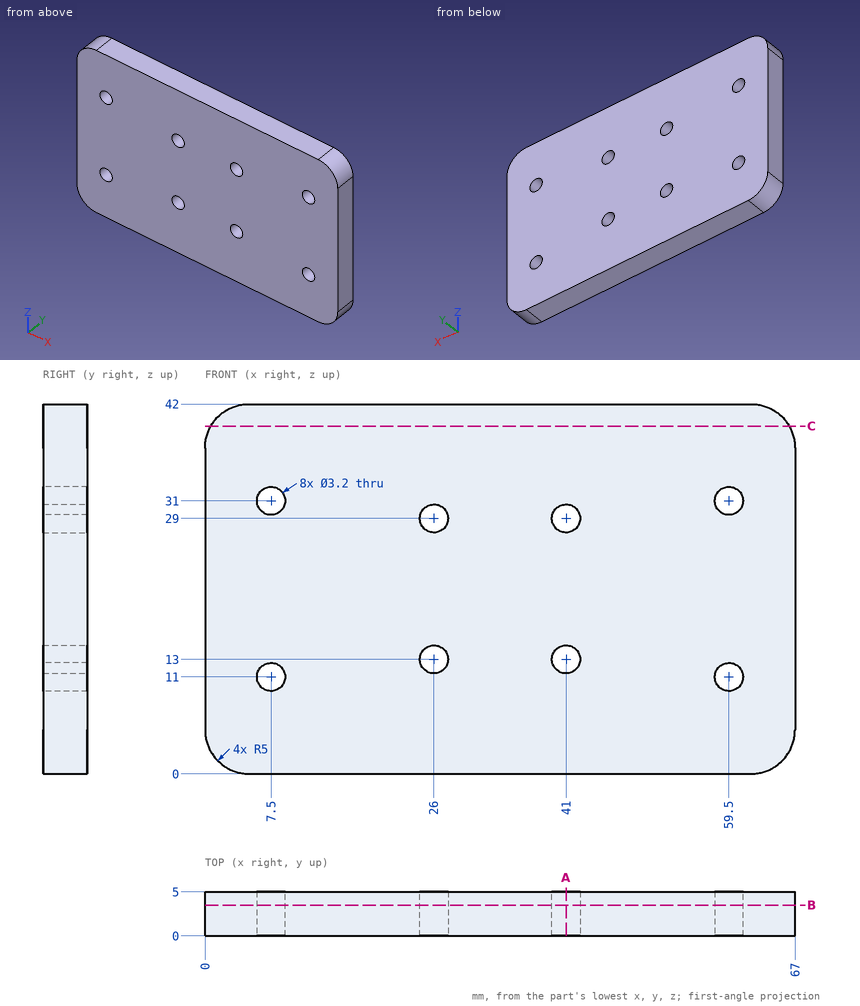
Study the drawing (mm; zero at the part's minimum x, y, z) and answer. Give positions to 0.01 mm unless a question says otherwise; leave off trailing zeros. Order: outer loops, then holes, each group sorted by start corner. A loop starts at its lowest first (then second) coordinate and runs counter-clockwise, first axis right, second up. Notation, with made-up numbers: M 67,41 L 109,41 A13 ccw 109,60 Z; hole C -25.5,84.5 d2. An arc over 180 degrees is marked long. Put each result on its own line as item: value. Start each with the question number.
Item 1: The part is cut by section A-A, the plane x = 41. Determine the outline of the cut face in (y, z).
Item 2: A flat-ended cylindrical pin translates along its axis: P1, Ø3, axis at x = 7.5, z = 11, coming from the +Y side. Find the tip coordinate at first contact, or state that the pin passes through.
Item 3: Find the intervals of material crossed by line 1 along Z through (x, y) = (59.5, 3.1); line 2 along X through (y, z) = (1.95, 13); line 3 along Z through (x, y) = (41, 2.55), in increasing order.
Item 4: The part is cut by section B-B, the plane y = 3.5. State how many separate pieces and enclosed holes the cut face has, and give its area (3 significant figures).
Item 5: The part is cut by section C-C, the plane z = 39.5. Determine the outline of the cut face in (x, y), and give its area (3 significant figures).
Answer key:
1. outline: M 0,0 L 5,0 L 5,11.4 L 0,11.4 Z; M 0,14.6 L 5,14.6 L 5,27.4 L 0,27.4 Z; M 0,30.6 L 5,30.6 L 5,42 L 0,42 Z
2. P1: passes through
3. line 1: z = 0 to 9.4, 12.6 to 29.4, 32.6 to 42
3. line 2: x = 0 to 24.4, 27.6 to 39.4, 42.6 to 67
3. line 3: z = 0 to 11.4, 14.6 to 27.4, 30.6 to 42
4. separate pieces: 1
4. enclosed holes: 8
4. area: 2,730 mm²
5. outline: M 0.67,0 L 66.33,0 L 66.33,5 L 0.67,5 Z
5. area: 328 mm²
